```python
from build123d import *

# Parameters (mm, degrees)
F0_W     = 50
F0_H     = 26
F1_DEPTH = 3
F2_W     = 50
F2_H     = 3
F3_DEPTH = 49
F4_R     = 2
F4_R_2   = 8.8
F5_DEPTH = 3
F6_R     = 5


with BuildPart() as f1:
    # F0 (on Top) → F1 (new body)
    with BuildSketch(Plane.XY):
        Polygon((25, 0), (0, 0), (-25, 0), (-25, -26), (25, -26), align=None)
        with BuildLine():
            ThreePointArc((-7.5, -12.5), (-7.93934, -13.56066), (-9, -14))
            Line((-9, -14), (-14, -14))
            ThreePointArc((-14, -14), (-15.06066, -13.56066), (-15.5, -12.5))
            Line((-15.5, -12.5), (-15.5, -11.5))
            ThreePointArc((-15.5, -11.5), (-15.06066, -10.43934), (-14, -10))
            Line((-14, -10), (-9, -10))
            ThreePointArc((-9, -10), (-7.93934, -10.43934), (-7.5, -11.5))
            Line((-7.5, -11.5), (-7.5, -12.5))
        make_face(mode=Mode.SUBTRACT)
        with BuildLine():
            Line((14, -14), (9, -14))
            ThreePointArc((9, -14), (7.93934, -13.56066), (7.5, -12.5))
            Line((7.5, -12.5), (7.5, -11.5))
            ThreePointArc((7.5, -11.5), (7.93934, -10.43934), (9, -10))
            Line((9, -10), (14, -10))
            ThreePointArc((14, -10), (15.06066, -10.43934), (15.5, -11.5))
            Line((15.5, -11.5), (15.5, -12.5))
            ThreePointArc((15.5, -12.5), (15.06066, -13.56066), (14, -14))
        make_face(mode=Mode.SUBTRACT)
        with Locations((0, -39)):
            Rectangle(F0_W, F0_H)
        with BuildLine():
            ThreePointArc((-7.5, -40.5), (-7.93934, -41.56066), (-9, -42))
            Line((-9, -42), (-14, -42))
            ThreePointArc((-14, -42), (-15.06066, -41.56066), (-15.5, -40.5))
            Line((-15.5, -40.5), (-15.5, -39.5))
            ThreePointArc((-15.5, -39.5), (-15.06066, -38.43934), (-14, -38))
            Line((-14, -38), (-9, -38))
            ThreePointArc((-9, -38), (-7.93934, -38.43934), (-7.5, -39.5))
            Line((-7.5, -39.5), (-7.5, -40.5))
        make_face(mode=Mode.SUBTRACT)
        with BuildLine():
            Line((15.5, -39.5), (15.5, -40.5))
            ThreePointArc((15.5, -40.5), (15.06066, -41.56066), (14, -42))
            Line((14, -42), (9, -42))
            ThreePointArc((9, -42), (7.93934, -41.56066), (7.5, -40.5))
            Line((7.5, -40.5), (7.5, -39.5))
            ThreePointArc((7.5, -39.5), (7.93934, -38.43934), (9, -38))
            Line((9, -38), (14, -38))
            ThreePointArc((14, -38), (15.06066, -38.43934), (15.5, -39.5))
        make_face(mode=Mode.SUBTRACT)
    extrude(amount=F1_DEPTH)

    # F2 (on face) → F3 (join)
    with BuildSketch(Plane.XY.offset(3)):
        with Locations((0, -1.5)):
            Rectangle(F2_W, F2_H)
    extrude(amount=F3_DEPTH)

    # F4 (on face) → F5 (cut)
    with BuildSketch(Plane(origin=(0, 0, 0), x_dir=(-1, 0, 0), z_dir=(0, 1, 0))):
        with Locations((-14.5, 28)):
            Circle(F4_R)
        with Locations((0, 28)):
            Circle(F4_R_2)
        with Locations((14.5, 28)):
            Circle(F4_R)
    extrude(amount=-F5_DEPTH, mode=Mode.SUBTRACT)

    # F6
    f6_edges = [f1.edges().sort_by_distance(p)[0] for p in [
        (-25, -1.5, 52),
        (25, -1.5, 52),
        (-25, -52, 1.5),
        (25, -52, 1.5),
    ]]
    fillet(f6_edges, radius=F6_R)


solid = f1.part
```
Geometry check sheet. Reference: the model listing, model coordinates, mm. A direction names the side the tool comes from. Coordinates: 2 decimals unless noted, no trailing zeros. Loops run counter-clockwise (first coordinate to the right, second up) from the corner with the lowest first, then second, coordinate; pieces in that order, holes last. Notation, with made-up numbers: (3.25, 71) - (32.25, 71) arc R23 cw to (32.25, 85) - close; hole circle Ø7 at (-33.5, 72). An arc over 180 degrees is marked (long way). One line per item, written item: value. Start each with the question number.
(1) Cross-section at C-C on y = -43.5. Enter the section's corners in (x, z), plus the area to 3 significant figures.
(2) Material ranges on line 1 (Z direction, x = 14.5, y = -0.9); line 2 (Z direction, x = -7, y = -33); line 3 (Z direction, x = 0, y = -0.95), recorded low to high. Write a range as [from, to].
(3) Tool access check on faces 1 (the flat face through (0, -3, 16)), 2 (the cylindrical face through (-15.05, -13.57, 1.48)), 3 (the cylindrical face through (23, -1, 51)). Record the directions out of +Z, -Z, +X, -X, +Y, -Y that give a thin tool (end or side, any length) a straight path to the whole face; none if there is none.
(4) Cross-section at B-B on x = 0. Enter the section's corners in (y, z), plus the area to 3 significant figures.
(5) Cross-section at A-A on z = 28. Enter the section's corners in (x, y).
(6) Depth check by flat-ended pin: P1, Ø12, axis at x = 10.5, z = 24.5, coming from the -Y side; P2, Ø10, axis at x = -6.5, y = -33, coming from the +Z side. Enter the tip coordinate at first touch or a pass-through.
(7) Cross-section at D-D on z = 22. Enter the section's corners in (x, y), plus the area to 3 significant figures.
(8) Mould release check, pull along Y, two halves, no side actions. Record for faces 4 (the cylindrical face through (-24, -50, 2)), 5 (the flat face through (-6, 0, 20)), 6 (the flat face through (11, -38, 1)), 7 (the flat face through (-25, -13.2, 2.5)): released by +Y, released by -Y, zero draft, split by the parting line, or undercut.
Results below:
1. outline: (-25, 0) - (25, 0) - (25, 3) - (-25, 3) - close
1. area: 150 mm2
2. line 1: z = [0, 26], [30, 52]
2. line 2: z = [0, 3]
2. line 3: z = [0, 19.2], [36.8, 52]
3. face 1: +Z, +X, -X, -Y
3. face 2: +Z, -Z
3. face 3: +Z, +X, +Y, -Y
4. outline: (-52, 0) - (0, 0) - (0, 19.2) - (-3, 19.2) - (-3, 3) - (-52, 3) - close; (-3, 36.8) - (0, 36.8) - (0, 52) - (-3, 52) - close
4. area: 250 mm2
5. outline: (-25, -3) - (-16.5, -3) - (-16.5, 0) - (-25, 0) - close; (-12.5, -3) - (-8.8, -3) - (-8.8, 0) - (-12.5, 0) - close; (8.8, -3) - (12.5, -3) - (12.5, 0) - (8.8, 0) - close; (16.5, -3) - (25, -3) - (25, 0) - (16.5, 0) - close
6. P1: stops at y = -3
6. P2: stops at z = 3
7. outline: (-25, -3) - (-6.44, -3) - (-6.44, 0) - (-25, 0) - close; (6.44, -3) - (25, -3) - (25, 0) - (6.44, 0) - close
7. area: 111 mm2
8. face 4: released by -Y
8. face 5: released by +Y
8. face 6: undercut
8. face 7: zero draft
